from build123d import *

# Parameters (mm, degrees)
CROQUIS1_R              = 1.1
FORMABASE_DEPTH         = 5
ESQUINAS_DEPTH          = 65.863317831
CROQUIS3_R              = 2
BARRENOSEJEZ_DEPTH      = 65.863317831
SALIENTE_EXTRUIR2_DEPTH = 5
CROQUIS5_R              = 2
CORTAR_EXTRUIR9_DEPTH   = 88.950270039


with BuildPart() as part:
    # Croquis1 → FormaBase (new body)
    with BuildSketch(Plane.XY):
        Polygon((20, 27.5), (-20, 27.5), (-20, -27.5), (-16, -31.5), (-16, -61.5), (16, -61.5), (16, -31.5), (20, -27.5), align=None)
        with Locations((-13.5, -32.5)):
            Circle(CROQUIS1_R, mode=Mode.SUBTRACT)
        with Locations((-13.5, -56.5)):
            Circle(CROQUIS1_R, mode=Mode.SUBTRACT)
        with Locations((13.5, -56.5)):
            Circle(CROQUIS1_R, mode=Mode.SUBTRACT)
        with Locations((13.5, -32.5)):
            Circle(CROQUIS1_R, mode=Mode.SUBTRACT)
    extrude(amount=FORMABASE_DEPTH)

    # Croquis2 → Esquinas (cut, through all)
    with BuildSketch(Plane.XY.offset(5)):
        Polygon((-20, 27.5), (-20, 23.497775618), (-15.997775618, 27.5), align=None)
        Polygon((20, 23.497775618), (15.997775618, 27.5), (20, 27.5), align=None)
    extrude(amount=-ESQUINAS_DEPTH, mode=Mode.SUBTRACT)

    # Croquis3 → BarrenosEjeZ (cut, through all)
    with BuildSketch(Plane.XY.offset(5)):
        with Locations((10.000556095, 10.499443905)):
            Circle(CROQUIS3_R)
        with Locations((10.000556095, -14.500556095)):
            Circle(CROQUIS3_R)
        with Locations(Location((-10.000556095, 10.499443905, 0), (0, 0, 180))):
            Circle(CROQUIS3_R)
        with Locations(Location((-10.000556095, -14.500556095, 0), (0, 0, 180))):
            Circle(CROQUIS3_R)
    extrude(amount=-BARRENOSEJEZ_DEPTH, mode=Mode.SUBTRACT)

    # Croquis4 → Saliente-Extruir2 (add, through all)
    with BuildSketch(Plane.XY.offset(5)):
        Polygon((-16, -61.5), (-16, -81.497775618), (-11.997775618, -85.5), (0, -85.5), (0, -61.5), align=None)
        Polygon((0, -61.5), (0, -85.5), (11.997775618, -85.5), (16, -81.497775618), (16, -61.5), align=None)
    extrude(amount=-SALIENTE_EXTRUIR2_DEPTH)

    # Croquis5 → Cortar-Extruir9 (cut, through all)
    with BuildSketch(Plane.XY.offset(5)):
        with Locations((0, -80.5)):
            Circle(CROQUIS5_R)
    extrude(amount=-CORTAR_EXTRUIR9_DEPTH, mode=Mode.SUBTRACT)


solid = part.part
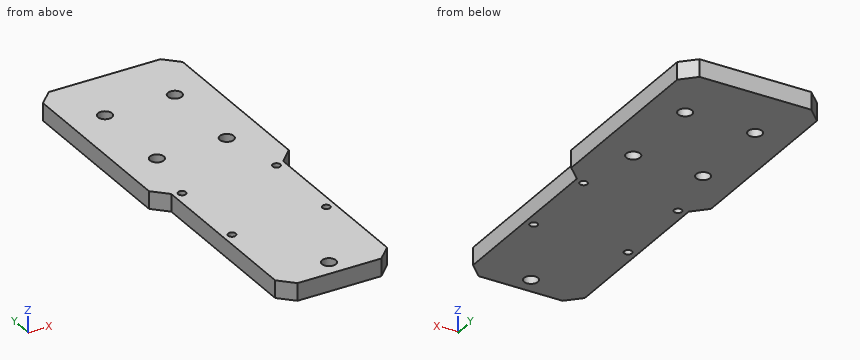
Design review of the part built by this model. Coordinates are the model's own, in mm. Round coordinates to 2 decimals unless told otherwise and drop trailing zeros. Order: outer loops, then holes, each group sorted by start corner. A loop starts at its lowest first (then second) coordinate and runs counter-clockwise, first axis right, second up. Notation, with made-up numbers: M -31,-30.75 L 19,-30.75 A5 cw 19,-21.75 Z; hole C 76,-36.5 d7. An arc over 180 degrees is marked long. Answer as CSV lines item,"result". Start each with the question number.
1) Add section A-A (y = -32.5). Give the boundary of the cut face in (x, z), then the cut area to 3 significant figures.
2) Add section D-D (x = -17). Give the boundary of the cut face in (y, z), then the cut area to 3 significant figures.
3) Add section B-B (x = 13.5). Give the boundary of the cut face in (y, z).
4) For pin 1 Ø6.5 at (x, y) = (0, -80.5) entering from -Z; pin 2 Ø2 at (y, z) = (-29, 2) entering from -X; pin 3 Ø1.5 at (y, z) = (-32, 0.5) entering from +X, all flat-tipped, find the tip position at first contact; note any pin that passes through.
5) Wall thickness on line 1 along Y through (x, z) = (0, 3.15); line 2 along Y through (x, z) = (-13.5, 3.7); line 3 along Y through (x, z) = (0.5, 4.65): over which ranges is each line inside the solid? List them lowest first. Write a range as [from, to].
6) Add section C-C (z = 3). Give the number of separate pieces and of enclosed holes in the cut face, then the cut area to 3 significant figures.
Resolved:
1,outline,"M -16,0 L -14.6,0 L -14.6,5 L -16,5 Z; M -12.4,0 L 12.4,0 L 12.4,5 L -12.4,5 Z; M 14.6,0 L 16,0 L 16,5 L 14.6,5 Z"
1,area,"138 mm^2"
2,outline,"M -30.5,0 L 26.5,0 L 26.5,5 L -30.5,5 Z"
2,area,"285 mm^2"
3,outline,"M -84,0 L -57.6,0 L -57.6,5 L -84,5 Z; M -55.4,0 L -33.6,0 L -33.6,5 L -55.4,5 Z; M -31.4,0 L 27.5,0 L 27.5,5 L -31.4,5 Z"
4,pin 1,"z = 0"
4,pin 2,"x = -19.5"
4,pin 3,"x = 16.25"
5,line 1,"[-85.5, -82.5], [-78.5, 27.5]"
5,line 2,"[-84, -57.6], [-55.4, -33.6], [-31.4, 27.5]"
5,line 3,"[-85.5, -82.44], [-78.56, 27.5]"
6,separate pieces,"1"
6,enclosed holes,"9"
6,area,"3,960 mm^2"
